Design review of the part built by this model. Coordinates are the model's own, in mm. Round coordinates to 2 decimals unless told otherwise and drop trailing zeros. Loops run counter-clockwise (first coordinate to the right, second up) from the corner with the lowest first, then second, coordinate; pieces in that order, holes last. Notation, with made-up numbers: (76, 45.25) - (101, 45.25) arc R23 cw to (101, 61.25) - close; hole circle Ø11 at (41.5, -31.5). An arc over 180 degrees is marked (long way). Return JSON: item names as keys, results as strings. Group by question number.
(1) We need section B-B, the plane y = -14. Write out the cut boundary in (x, z).
(2) Clearance check with flat-ended pins moving along their axes: pin 1 (1.8 mm diameter, centred on x = -40, y = 35, fed in from +Z); pin 2 (1 mm diameter, centred on y = 41, z = 1.5, fed in from -X). State where each tip first meets the part, or that it passes through.
(3) We need section C-C, the plane x = -46. Write out the cut boundary in (y, z).
(4) We need section A-A, the plane z = 0.8. Give the number of separate pieces and of enclosed holes in the cut face, and give its area (3 significant figures).
(5) Wall thickness on L1, parallel to Y at x = 25, z = 1.4; L2, parallel to Y at x = -40, z = 0.45; L3, parallel to X at y = 10, z = 1.25: over which ranges is each line inside the solid? List them lowest first. Write a range as [from, to].
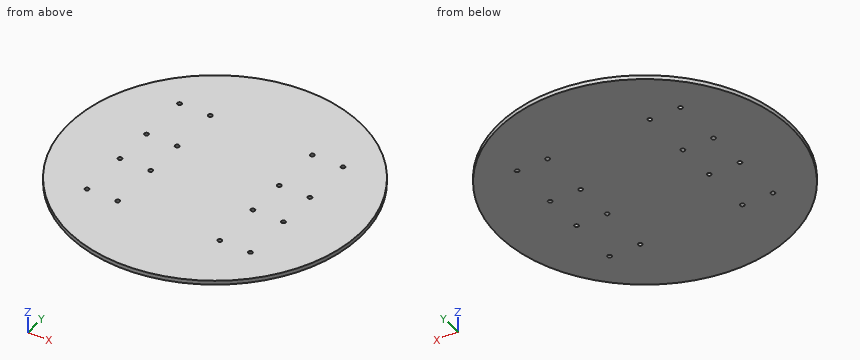
from build123d import *

# Parameters (mm, degrees)
SKETCH_1_R               = 70.710678119
EXTRUDE_1_DEPTH          = 2
SKETCH_2_R               = 1
CUT_EXTRUDE_4_DEPTH      = 101.019998
MIRROR_6_COPY_1_SKETCH_R = 1
MIRROR_6_COPY_1_DEPTH    = 101.019998


with BuildPart() as part:
    # ｽｹｯﾁ1 → ﾎﾞｽ - 押し出し1 (new body)
    with BuildSketch(Plane.XY):
        Circle(SKETCH_1_R)
    extrude(amount=EXTRUDE_1_DEPTH)

    # ｽｹｯﾁ2 → ｶｯﾄ - 押し出し4 (cut, symmetric)
    with BuildSketch(Plane.XY):
        with Locations((25, -10)):
            Circle(SKETCH_2_R)
        with Locations((40, -10)):
            Circle(SKETCH_2_R)
        with Locations((25, -35)):
            Circle(SKETCH_2_R)
        with Locations((40, -35)):
            Circle(SKETCH_2_R)
    cut_extrude_4 = extrude(amount=CUT_EXTRUDE_4_DEPTH, both=True, mode=Mode.SUBTRACT)

    # ﾐﾗｰ2: ｶｯﾄ - 押し出し4 across plane
    add(cut_extrude_4.mirror(Plane(origin=(0, 0, 0), x_dir=(0, 0, 1), z_dir=(1, 0, 0))), mode=Mode.SUBTRACT)

    # ﾐﾗｰ6: ｶｯﾄ - 押し出し4 across plane
    add(cut_extrude_4.mirror(Plane.ZX), mode=Mode.SUBTRACT)

    # ﾐﾗｰ6 copy 1 sketch → ﾐﾗｰ6 copy 1 (cut, symmetric)
    with BuildSketch(Plane(origin=(0, 0, 0), x_dir=(-1, 0, 0), z_dir=(0, 0, 1))):
        with Locations((25, -10)):
            Circle(MIRROR_6_COPY_1_SKETCH_R)
        with Locations((40, -10)):
            Circle(MIRROR_6_COPY_1_SKETCH_R)
        with Locations((25, -35)):
            Circle(MIRROR_6_COPY_1_SKETCH_R)
        with Locations((40, -35)):
            Circle(MIRROR_6_COPY_1_SKETCH_R)
    extrude(amount=MIRROR_6_COPY_1_DEPTH, both=True, mode=Mode.SUBTRACT)


solid = part.part
Solutions:
{
 "1": {"outline": "(-69.31, 0) - (69.31, 0) - (69.31, 2) - (-69.31, 2) - close"},
 "2": {"pin 1": "through", "pin 2": "x = -57.96"},
 "3": {"outline": "(-53.7, 0) - (53.7, 0) - (53.7, 2) - (-53.7, 2) - close"},
 "4": {"separate pieces": "1", "enclosed holes": "16", "area": "15,700 mm^2"},
 "5": {"L1": "[-66.14, -36], [-34, -11], [-9, 9], [11, 34], [36, 66.14]", "L2": "[-58.31, -36], [-34, -11], [-9, 9], [11, 34], [36, 58.31]", "L3": "[-70, -41], [-39, -26], [-24, 24], [26, 39], [41, 70]"}
}
